Verification items for the finished model (mm, model axes). Face numbers are marked on the shaded views. A direction names the side the tool comes from. Round coordinates to 2 decimals unless told otherwise and drop trailing zeros. Write each loop counter-clockwise with the first axis right and the second up, starting at its lowest first coordinate (ties: lowest second). Pieces come first, ordered by that corner, then holes. Notation, with made-up numbers: M 45,33 L 64,33 A26 cw 64,61 Z; hole C -23,-12 d8. An arc over 180 degrees is marked long. One line per item, written item: value. Start each with the question number.
Item 1: Gauge pin test, flat ends, axial feed: pin 1 (12.5 mm diameter, centred on y = 2, z = 41, fed in from -X); pin 2 (4.5 mm diameter, centred on y = 2, z = 42.5, fed in from +X); pin 3 (1 mm diameter, centred on y = 71, z = 181, fed in from -X); pin 4 (10 mm diameter, centred on x = 2, y = -30.5, fed in from -Z). Record the tip position at first contact, or that the pin passes through.
Item 2: Section check D-D, the plane z = 237.5. Record the cut outline in (x, y), then the cut area to 3 significant figures.
Item 3: Thickness scan on probe 1 along Y at (x, z) = (0, 279); probe 2 along Z at (x, y) = (-71.5, 30.5); probe 3 along Y at (x, z) = (-10, 256). Record the ranges inside material, lowest first. Write a range as from..to.
Item 4: Draft check along Y on the marked faces 3, 4 and 5. Enter one of: +Y half, -Y half, draft (parallel to the pull), parting line (faces both ways), or undercut.
Item 5: Section check B-B, the plane z = 63. Record the cut outline in (x, y).
Item 6: Section check A-A, the plane y = 0. Record the cut outline in (x, z), then the cut area to 3 significant figures.
Item 7: Tool access check on the marked faces 1 and 2. Record the directions out of +Z, -Z, +X, -X, +Y, -Y that give a thin tool (end or side, any length) a straight path to the whole face; none if there is none.
from build123d import *

# Parameters (mm, degrees)
F0_R     = 38.1
F1_DEPTH = 101.6
F2_R     = 101.6
F2_R_2   = 38.1
F3_DEPTH = 203.2
F4_R     = 25.4
F5_DEPTH = 50.8


with BuildPart() as f1:
    # F0 (on Top) → F1 (new body)
    with BuildSketch(Plane.XY):
        Circle(F0_R)
        Polygon((-19.05, 7.890768), (-7.890768, 19.05), (7.890768, 19.05), (19.05, 7.890768), (19.05, -7.890768), (7.890768, -19.05), (-7.890768, -19.05), (-19.05, -7.890768), align=None, mode=Mode.SUBTRACT)
    extrude(amount=F1_DEPTH)

    # F2 (on face) → F3 (join)
    with BuildSketch(Plane.XY.offset(101.6)):
        Circle(F2_R)
        Circle(F2_R_2, mode=Mode.SUBTRACT)
        Circle(F2_R)
    extrude(amount=F3_DEPTH)

    # F4 (on face) → F5 (cut)
    with BuildSketch(Plane.XY.offset(304.8)):
        Circle(F4_R)
    extrude(amount=-F5_DEPTH, mode=Mode.SUBTRACT)


solid = f1.part
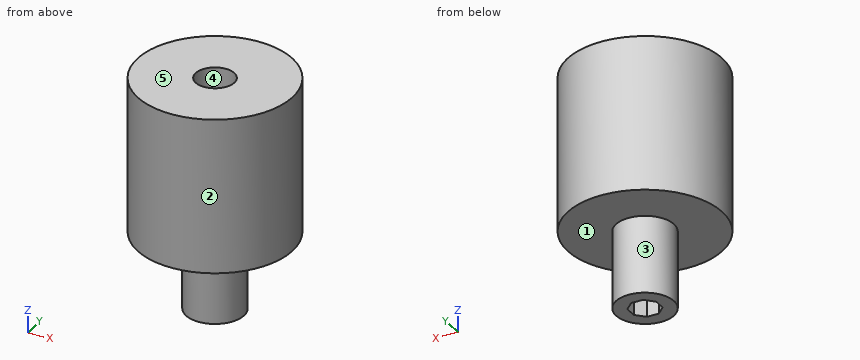
Response values:
1. pin 1: stops at x = -38.1
1. pin 2: stops at x = 38.1
1. pin 3: stops at x = -73.16
1. pin 4: stops at z = 0
2. outline: C 0,0 d203.2
2. area: 32,400 mm2
3. probe 1: y = -101.6..-25.4, 25.4..101.6
3. probe 2: z = 101.6..304.8
3. probe 3: y = -101.11..-23.35, 23.35..101.11
4. face 3: parting line
4. face 4: undercut
4. face 5: draft
5. outline: C 0,0 d76.2; hole M -19.05,-7.89 L -7.89,-19.05 L 7.89,-19.05 L 19.05,-7.89 L 19.05,7.89 L 7.89,19.05 L -7.89,19.05 L -19.05,7.89 Z
6. outline: M -101.6,101.6 L -38.1,101.6 L -38.1,0 L -19.05,0 L -19.05,101.6 L 19.05,101.6 L 19.05,0 L 38.1,0 L 38.1,101.6 L 101.6,101.6 L 101.6,304.8 L 25.4,304.8 L 25.4,254 L -25.4,254 L -25.4,304.8 L -101.6,304.8 Z
6. area: 42,600 mm2
7. face 1: -Z
7. face 2: +Z, -Z
